For this review, take the finished solid that the model builds, in its own axes (mm). A direction names the side the tool comes from. Give positions to 0.01 mm unless a question says otherwise; leave off trailing zeros. Loops run counter-clockwise (first coordinate to the right, second up) from the corner with the lowest first, then second, coordinate; pieces in that order, holes last. Notation, with made-up numbers: (12, 68) - (64, 68) arc R27 cw to (64, 100) - close; hole circle Ø5 at (84.25, -29). An arc over 180 degrees is marked (long way). Put each result on its own line as item: value. Start each with the question number.
from build123d import *

# Parameters (mm, degrees)
TOP_COVER_SKETCH_01_W       = 44.37
TOP_COVER_SKETCH_01_H       = 23.06
TOP_COVER_EXT_SHAPE_DEPTH   = 4.3
SALIENTE_EXTRUIR1_DEPTH     = 1.5
VACIADO1_T                  = -1
VACIADO1_THICKNESS_2_FACE_W = 21.06
VACIADO1_THICKNESS_2_FACE_H = 3.3
VACIADO1_THICKNESS_2_DEPTH  = 0.31
VACIADO1_THICKNESS_3_FACE_W = 21.06
VACIADO1_THICKNESS_3_FACE_H = 3.3
VACIADO1_THICKNESS_3_DEPTH  = 0.31
VACIADO1_THICKNESS_4_FACE_W = 42.99
VACIADO1_THICKNESS_4_FACE_H = 3.3
VACIADO1_THICKNESS_4_DEPTH  = 0.02
VACIADO1_THICKNESS_5_FACE_W = 42.99
VACIADO1_THICKNESS_5_FACE_H = 3.3
VACIADO1_THICKNESS_5_DEPTH  = 0.3
CROQUIS1_R                  = 3.25
CORTAR_EXTRUIR1_DEPTH       = 0.7
CROQUIS1_5_R                = 5
CROQUIS1_5_R_2              = 3.25
CORTAR_EXTRUIR2_DEPTH       = 0.5
CROQUIS2_R                  = 3
SALIENTE_EXTRUIR2_DEPTH     = 3.7
REDONDEO1_R                 = 0.5
REDONDEO2_R                 = 0.3
TOP_COVER_SKETCH_01_19_R    = 0.85
CORTAR_EXTRUIR3_DEPTH       = 1


with BuildPart() as part:
    # Top-cover-sketch-01 → Top-cover-ext-shape (new body)
    with BuildSketch(Plane(origin=(0, 0, 0), x_dir=(1, 0, 0), z_dir=(0, 1, 0))):
        Rectangle(TOP_COVER_SKETCH_01_W, TOP_COVER_SKETCH_01_H)
    extrude(amount=TOP_COVER_EXT_SHAPE_DEPTH)

    # Top-cover-sketch-01<18> → Saliente-Extruir1 (add)
    with BuildSketch(Plane(origin=(0, 0, 0), x_dir=(1, 0, 0), z_dir=(0, 1, 0))):
        with BuildLine():
            Line((-19.255, -4.986911136), (-19.255, 4.986911136))
            ThreePointArc((-19.255, 4.986911136), (-17.190017633, 6.076280801), (-16.025784389, 8.1))
            Line((-16.025784389, 8.1), (16.025784389, 8.1))
            ThreePointArc((16.025784389, 8.1), (17.190017633, 6.076280801), (19.255, 4.986911136))
            Line((19.255, 4.986911136), (19.255, -4.986911136))
            ThreePointArc((19.255, -4.986911136), (17.190017633, -6.076280801), (16.025784389, -8.1))
            Line((16.025784389, -8.1), (-16.025784389, -8.1))
            ThreePointArc((-16.025784389, -8.1), (-17.190017633, -6.076280801), (-19.255, -4.986911136))
        make_face()
    extrude(amount=-SALIENTE_EXTRUIR1_DEPTH)

    # Vaciado1
    vaciado1_openings = [part.faces().sort_by_distance(p)[0] for p in [
        (0, 4.3, 0),
    ]]
    offset(amount=VACIADO1_T, openings=vaciado1_openings, kind=Kind.INTERSECTION)

    # Vaciado1 thickness 2 face (on inner face of the shell) → Vaciado1 thickness 2 (cut)
    with BuildSketch(Plane(origin=(-21.185, 2.65, 0), x_dir=(0, 0, -1), z_dir=(-1, 0, 0))):
        Rectangle(VACIADO1_THICKNESS_2_FACE_W, VACIADO1_THICKNESS_2_FACE_H)
    extrude(amount=VACIADO1_THICKNESS_2_DEPTH, mode=Mode.SUBTRACT)

    # Vaciado1 thickness 3 face (on inner face of the shell) → Vaciado1 thickness 3 (cut)
    with BuildSketch(Plane(origin=(21.185, 2.65, 0), x_dir=(0, 0, 1), z_dir=(1, 0, 0))):
        Rectangle(VACIADO1_THICKNESS_3_FACE_W, VACIADO1_THICKNESS_3_FACE_H)
    extrude(amount=VACIADO1_THICKNESS_3_DEPTH, mode=Mode.SUBTRACT)

    # Vaciado1 thickness 4 face (on inner face of the shell) → Vaciado1 thickness 4 (cut)
    with BuildSketch(Plane(origin=(0, 2.65, -10.53), x_dir=(-1, 0, 0), z_dir=(0, 0, -1))):
        Rectangle(VACIADO1_THICKNESS_4_FACE_W, VACIADO1_THICKNESS_4_FACE_H)
    extrude(amount=VACIADO1_THICKNESS_4_DEPTH, mode=Mode.SUBTRACT)

    # Vaciado1 thickness 5 face (on inner face of the shell) → Vaciado1 thickness 5 (add)
    with BuildSketch(Plane(origin=(0, 2.65, 10.53), x_dir=(1, 0, 0), z_dir=(0, 0, 1))):
        Rectangle(VACIADO1_THICKNESS_5_FACE_W, VACIADO1_THICKNESS_5_FACE_H)
    extrude(amount=-VACIADO1_THICKNESS_5_DEPTH)

    # Croquis1 → Cortar-Extruir1 (cut)
    with BuildSketch(Plane.XZ.offset(1.5)):
        with Locations(Location((-11.878900962, 0, 0), (0, 0, 270))):
            Circle(CROQUIS1_R)
    extrude(amount=-CORTAR_EXTRUIR1_DEPTH, mode=Mode.SUBTRACT)

    # Croquis1<5> → Cortar-Extruir2 (cut)
    with BuildSketch(Plane.XZ.offset(1.5)):
        with Locations(Location((-11.878900962, 0, 0), (0, 0, 270))):
            Circle(CROQUIS1_5_R)
        with Locations(Location((-11.878900962, 0, 0), (0, 0, 270))):
            Circle(CROQUIS1_5_R_2, mode=Mode.SUBTRACT)
    extrude(amount=-CORTAR_EXTRUIR2_DEPTH, mode=Mode.SUBTRACT)

    # Croquis2 → Saliente-Extruir2 (add)
    with BuildSketch(Plane.XZ.offset(0.8)):
        with Locations(Location((-11.878900962, 0, 0), (0, 0, 270))):
            Circle(CROQUIS2_R)
    extrude(amount=SALIENTE_EXTRUIR2_DEPTH)

    # Redondeo1
    redondeo1_edges = [part.edges().sort_by_distance(p)[0] for p in [
        (0, 0, -11.53),
        (22.185, 0, 0),
        (0, 0, 11.53),
        (-22.185, 0, 0),
        (-22.185, 2.15, -11.53),
        (22.185, 2.15, -11.53),
        (22.185, 2.15, 11.53),
        (-22.185, 2.15, 11.53),
    ]]
    fillet(redondeo1_edges, radius=REDONDEO1_R)

    # Redondeo2
    redondeo2_edges = [part.edges().sort_by_distance(p)[0] for p in [
        (-19.255, -0.75, 4.986911136),
        (-19.255, -0.75, -4.986911136),
        (-16.025784389, -0.75, -8.1),
        (16.025784389, -0.75, -8.1),
        (19.255, -0.75, -4.986911136),
        (19.255, -0.75, 4.986911136),
        (0, -1.5, 8.1),
        (16.025784389, -0.75, 8.1),
        (-17.190017633, -1.5, 6.076280801),
        (-16.025784389, -0.75, 8.1),
        (-19.255, -1.5, 0),
        (-17.190017633, -1.5, -6.076280801),
        (0, -1.5, -8.1),
        (17.190017633, -1.5, -6.076280801),
        (19.255, -1.5, 0),
        (17.190017633, -1.5, 6.076280801),
        (-11.878900962, -1.5, 5),
    ]]
    fillet(redondeo2_edges, radius=REDONDEO2_R)

    # Chaflán1: read off the stored shape, not the designer's step
    # Chaflán1 outline → Chaflán1 (revolve, cut)
    with BuildSketch(Plane(origin=(-11.878900962, 0, 0), x_dir=(1, 0, 0), z_dir=(0, 0, 1))):
        Polygon((3, -4.2), (2.7, -4.5), (3, -4.5), align=None)
    revolve(axis=Axis((-11.878900962, 0, 0), (0, 1, 0)), mode=Mode.SUBTRACT)

    # Top-cover-sketch-01<19> → Cortar-Extruir3 (cut)
    with BuildSketch(Plane(origin=(0, 0, 0), x_dir=(1, 0, 0), z_dir=(0, 1, 0))):
        with Locations(Location((-20.105, 9.1, 0), (0, 0, 270))):
            Circle(TOP_COVER_SKETCH_01_19_R)
        with Locations(Location((20.105, 9.1, 0), (0, 0, 270))):
            Circle(TOP_COVER_SKETCH_01_19_R)
        with Locations(Location((20.105, -9.1, 0), (0, 0, 270))):
            Circle(TOP_COVER_SKETCH_01_19_R)
        with Locations(Location((-20.105, -9.1, 0), (0, 0, 270))):
            Circle(TOP_COVER_SKETCH_01_19_R)
    extrude(amount=CORTAR_EXTRUIR3_DEPTH, mode=Mode.SUBTRACT)


solid = part.part
1) Take a section at B-B on y = 3.5. State the section outline as (x, z) points (3 decimals), and give its area (3 significant figures).
2) Mouldability with a two-part tool opening along X and no side actions: class faces 1 (the cylindrical face through (-20.86, 0.49, 9.49)), 2 (the cylindrical face through (-17.209, -0.592, -6.058)), 3 (the cylindrical face through (20.679, 0.493, -9.726)), 4 (the flat face through (22.185, 2, 0)) as released by +X, released by -X, zero draft, split by the parting line, or undercut.
3) Wall thickness on probe 1 along Z at (x, y) = (3.5, 1.5); probe 2 along X at (y, z) = (2.5, 9.75) (3 decimals); probe 3 along Z at (x, y) = (-14.5, 0.5): over which ranges is each line inside the solid? List them lowest first.
4) Take a section at D-D on y = -2.25. State the section outline as (x, z) points, and give its area (3 significant figures).
5) Take a section at C-C on x = 11.5. State the section outline as (y, z) points.
6) Take a section at A-A on z = -9.1. State the section outline as (x, y) points (3 decimals), and give its area (3 significant figures).
7) Machinability: for faces 5 (the cylindrical face through (17.209, -0.592, 6.058)), 6 (the flat face through (18.255, 0, 0)), 7 (the cylindrical face through (-17.166, -0.592, 6.1)), 8 (the flat face through (-19.255, -1, 0)), 9 (the flat face through (-15.14, -1, -1.04)), which of the approach directions +Z, -Z, +X, -X, +Y, -Y give a long, thin tool a straight path to every point of the face, cutting with its end or side? Answer none if there is none.
8) Insertion check: P1, Ø1, axis at x = -12.5, z = 6.5, coming from the +Y side; P2, Ø4, axis at x = -2, z = 3, coming from the -Y side; P3, Ø3, axis at x = 17, z = -2, coming from the +Y side. Each pin has a flat end and moves straight along its axis. Give the tip position at first contact, or say it passes through.
Answers follow:
1. outline: (-22.185, -11.03) arc R0.5 ccw to (-21.685, -11.53) - (21.685, -11.53) arc R0.5 ccw to (22.185, -11.03) - (22.185, 11.03) arc R0.5 ccw to (21.685, 11.53) - (-21.685, 11.53) arc R0.5 ccw to (-22.185, 11.03) - close; hole (-21.495, -10.55) - (21.495, -10.55) - (21.495, 10.23) - (-21.495, 10.23) - close
1. area: 130 mm2
2. face 1: undercut
2. face 2: released by -X
2. face 3: undercut
2. face 4: released by +X
3. probe 1: -11.53 to -10.55, 10.23 to 11.53
3. probe 2: -22.185 to -21.495, 21.495 to 22.185
3. probe 3: -11.53 to -7.1, 7.1 to 11.53
4. outline: circle Ø6 at (-11.88, 0)
4. area: 28.3 mm2
5. outline: (-1.5, -7.8) arc R0.3 ccw to (-1.2, -8.1) - (0, -8.1) - (0, -11.03) arc R0.5 ccw to (0.5, -11.53) - (4.3, -11.53) - (4.3, -10.55) - (1, -10.55) - (1, -7.1) - (-0.5, -7.1) - (-0.5, 7.1) - (1, 7.1) - (1, 10.23) - (4.3, 10.23) - (4.3, 11.53) - (0.5, 11.53) arc R0.5 ccw to (0, 11.03) - (0, 8.1) - (-1.2, 8.1) arc R0.3 ccw to (-1.5, 7.8) - close
6. outline: (-22.185, 0.5) arc R0.5 ccw to (-21.685, 0) - (-20.955, 0) - (-20.955, 1) - (-21.495, 1) - (-21.495, 4.3) - (-22.185, 4.3) - close; (-19.255, 0) - (19.255, 0) - (19.255, 1) - (-19.255, 1) - close; (20.955, 0) - (21.685, 0) arc R0.5 ccw to (22.185, 0.5) - (22.185, 4.3) - (21.495, 4.3) - (21.495, 1) - (20.955, 1) - close
6. area: 45.4 mm2
7. face 5: +Z, +X, -Y
7. face 6: +Y
7. face 7: +Z, -X, -Y
7. face 8: +Z, -Z, -X, -Y
7. face 9: -Y
8. P1: y = -0.5
8. P2: y = -1.5
8. P3: y = 1
